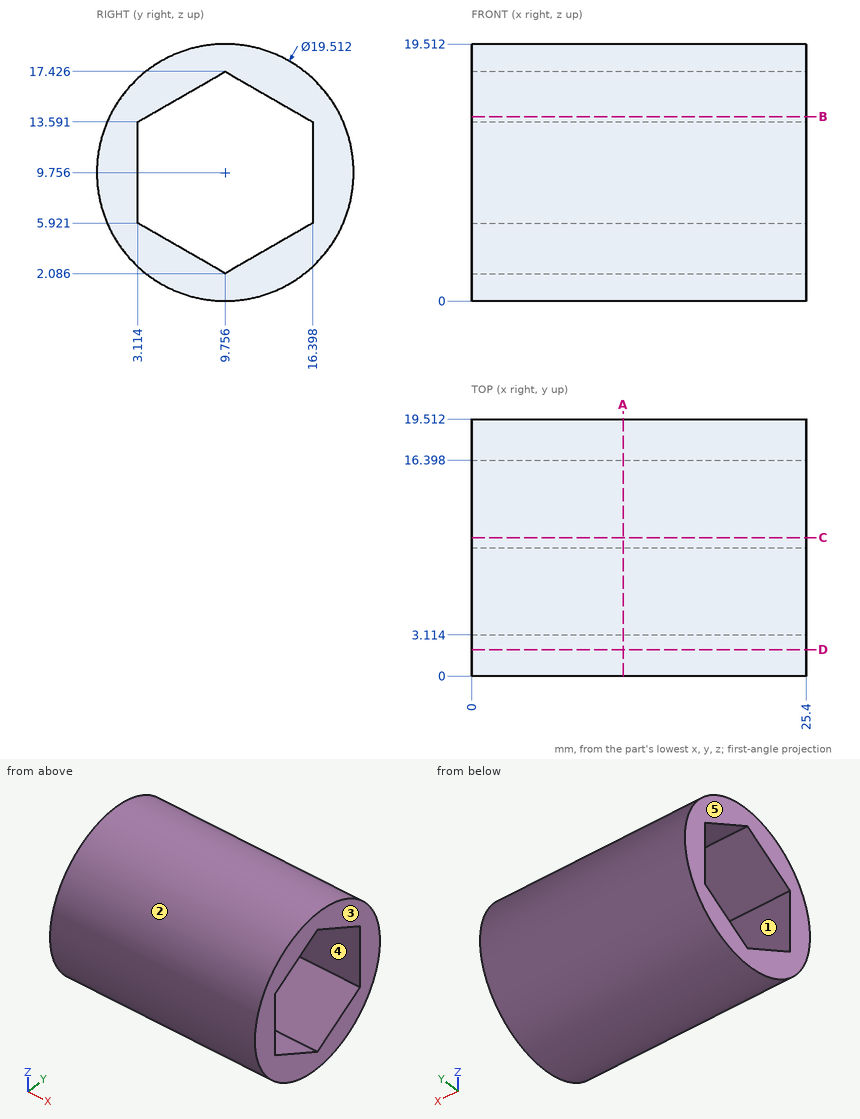
Can you work these out from the drawing? Everything is in mm from the part's minimum corner. A direction names the side the tool comes from. Coordinates: 2 decimals unless noted, no trailing zeros. Loops run counter-clockwise (first coordinate to the right, second up) from the corner with the lowest first, then second, coordinate; pieces in that order, holes last. Notation, with made-up numbers: (83, 17) - (132, 17) arc R14 cw to (132, 34) - close; hole circle Ø7 at (-15, 13.25). An arc over 180 degrees is marked (long way). Use a Markdown table: item, result.
Item 1: I want a section at D-D on y = 2. Please give me the cut outline in (x, z).
Numbers:
| item | result |
|---|---|
| outline | (0, 3.84) - (25.4, 3.84) - (25.4, 15.67) - (0, 15.67) - close |
Item 2: We'd pull the mould along Y, two halves only. Please class the marked faces 1, 2 and 3: released by +Y, released by -Y, zero draft, split by the parting line, or undercut.
Numbers:
| item | result |
|---|---|
| face 1 | undercut |
| face 2 | split by the parting line |
| face 3 | zero draft |
Item 3: I want a section at A-A on x = 11.5. Please give me the cut outline in (y, z) (1 decimal), and give its area (3 significant figures).
Numbers:
| item | result |
|---|---|
| outline | circle Ø19.5 at (9.8, 9.8); hole (3.1, 5.9) - (9.8, 2.1) - (16.4, 5.9) - (16.4, 13.6) - (9.8, 17.4) - (3.1, 13.6) - close |
| area | 146 mm2 |
Item 4: Will these pins go through, and if not, where does the flat tip stop? pin 1 (8.5 mm diameter, centred on x = 14.5, z = 11.5, fed in from +Y); pin 2 (2 mm diameter, centred on x = 18.5, z = 2.5, fed in from -Y); pin 3 (1 mm diameter, centred on x = 20.5, y = 6, fed in from +Z); pin 4 (1.5 mm diameter, centred on x = 10.5, z = 2.5, fed in from -Y) (1 decimal).
Numbers:
| item | result |
|---|---|
| pin 1 | stops at y = 19.51 |
| pin 2 | stops at y = 2.27 |
| pin 3 | stops at z = 18.95 |
| pin 4 | stops at y = 2.5 |
Item 5: I want a section at C-C on y = 10.5. Please give me the cut outline in (x, z), and give its area (3 significant figures).
Numbers:
| item | result |
|---|---|
| outline | (0, 0.03) - (25.4, 0.03) - (25.4, 2.52) - (0, 2.52) - close; (0, 17) - (25.4, 17) - (25.4, 19.48) - (0, 19.48) - close |
| area | 126 mm2 |
Item 6: If I drill on probe 1 along Y at (x, z) = (10, 10); probe 2 along Y at (x, z) = (20.25, 5.75); probe 3 along Z at (x, y) = (10.75, 8), over which ranges is the centre line in solid material (lowest first)? Write a range as from..to.
Numbers:
| item | result |
|---|---|
| probe 1 | y = 0..3.11, 16.4..19.51 |
| probe 2 | y = 0.86..3.41, 16.1..18.65 |
| probe 3 | z = 0.16..3.1, 16.41..19.35 |
Item 7: I want a section at B-B on z = 14. Please give me the cut outline in (x, y).
Numbers:
| item | result |
|---|---|
| outline | (0, 0.97) - (25.4, 0.97) - (25.4, 3.82) - (0, 3.82) - close; (0, 15.69) - (25.4, 15.69) - (25.4, 18.54) - (0, 18.54) - close |
Item 8: For the marked faces 4 and 5, which set-ups out of +Z, -Z, +X, -X, +Y, -Y let a thin tool reach every point of the face, with its end or its side?
Numbers:
| item | result |
|---|---|
| face 4 | +X, -X |
| face 5 | +Z, -Z, -X, +Y, -Y |
